Geometry check sheet. Reference: the model listing, model coordinates, mm. A direction names the side the tool comes from. Give positions to 0.01 mm unless a question says otherwise; leave off trailing zeros. Order: outer loops, then holes, each group sorted by start corner. A loop starts at its lowest first (then second) coordinate and runs counter-clockwise, first axis right, second up. Notation, with made-up numbers: (75, 1) - (107, 1) arc R22 ccw to (107, 21) - close; hole circle Ø7 at (29.25, 61). An arc over 180 degrees is marked (long way). Put each result on its own line as item: value. Start each with the question number.
Autodesk Inventor part; units mm, degrees
ref_plane "YZ Plane" through (0, 0, 0) normal (1, 0, 0) x (0, 1, 0)
ref_plane "XZ Plane" through (0, 0, 0) normal (0, 1, 0) x (-1, 0, 0)
ref_plane "XY Plane" through (0, 0, 0) normal (0, 0, 1) x (1, 0, 0)
sketch "Skizze1" plane through (0, 0, 0) normal (0, 0, 1) x (1, 0, 0)
  line L0 (-5.6, 0) -> (5.6, 0)
  line L1 (0, -5.6) -> (0, 5.6)
  circle A0 centre (0, 0) radius 4
  dimension "d0" = 8
extrude "Extrusion1" add sketch "Skizze1" along normal blind 10
sketch "Skizze2" plane through (0, 0, 0) normal (0, 0, -1) x (-1, 0, 0)
  circle A0 centre (0, 0) radius 3
  dimension "d3" = 6
extrude "Extrusion2" add sketch "Skizze2" along normal blind 6
sketch "Skizze3" plane through (0, 0, -6) normal (0, 0, -1) x (-1, 0, 0)
  circle A0 centre (0, 0) radius 2.5
  dimension "d6" = 5
extrude "Extrusion3" add sketch "Skizze3" along normal blind 1
sketch "Skizze4" plane through (0, 0, -7) normal (0, 0, -1) x (-1, 0, 0)
  circle A0 centre (0, 0) radius 3
extrude "Extrusion4" add sketch "Skizze4" along normal blind 3
sketch "Skizze5" plane through (0, 0, 10) normal (0, 0, 1) x (1, 0, 0)
  circle A0 centre (0, 0) radius 0.5
  dimension "d11" = 1
extrude "Extrusion5" cut sketch "Skizze5" against normal blind 20
chamfer "Fase1" distance 0.5 angle 45 1 edges at (-4, 0, 10)
properties part number "Nebeldüse"
Item 1: Cross-section at D-D (z = 6.75). Enter the section's corners in (x, y), and give its area (3 significant figures).
Item 2: Release check for a two-part mould opening along Z. For faces 4 (the face through (0, -1, 10)), 5 (the face through (-1, 0, -10)), 6 (the face through (0.54, 2.44, -6.49)) record: +Z half, -Z half, draft (parallel to the pull), parting line (faces both ways), or undercut.
Item 3: Thickness scan on line 1 along Z through (x, y) = (2, 2); line 2 along Z through (x, y) = (2, -2.5); line 3 along Y through (x, z) = (-2.75, -7.5). Record the ranges inside material, lowest first.
Item 4: Cross-section at C-C (z = -1). Enter the section's corners in (x, y).
Item 5: Set-up check for faces 1 (the face through (-0.867, 3.905, 4.684)), 2 (the face through (2, 2, -6)), 3 (the face through (3, 0, -8)): record each of +Z, -Z, +X, -X, +Y, -Y from which the full face is reachable in a straight line by a thin tool's end or side.
Item 6: Cross-section at A-A (y = 0). Enter the section's corners in (x, z).
Item 7: Gauge pin test, flat ends, axial feed: pin 1 Ø1 at (y, z) = (1.5, -6) entering from +X; pin 2 Ø1.5 at (x, z) = (-2, -3.5) entering from -Y. Record the tip position at first contact, or that the pin passes through.
Recorded:
1. outline: circle Ø8 at (0, 0); hole circle Ø1 at (0, 0)
1. area: 49.5 mm^2
2. face 4: +Z half
2. face 5: -Z half
2. face 6: undercut
3. line 1: z = -10 to -7, -6 to 10
3. line 2: z = 0 to 10
3. line 3: y = -1.2 to 1.2
4. outline: circle Ø6 at (0, 0); hole circle Ø1 at (0, 0)
5. face 1: +Z, -Z
5. face 2: none
5. face 3: -Z
6. outline: (-4, 0) - (-3, 0) - (-3, -6) - (-2.5, -6) - (-2.5, -7) - (-3, -7) - (-3, -10) - (-0.5, -10) - (-0.5, 10) - (-3.5, 10) - (-4, 9.5) - close; (0.5, -10) - (3, -10) - (3, -7) - (2.5, -7) - (2.5, -6) - (3, -6) - (3, 0) - (4, 0) - (4, 9.5) - (3.5, 10) - (0.5, 10) - close
7. pin 1: stops at x = 2.83
7. pin 2: stops at y = -2.73
